Print and shaded views of the part. All mm, measured from the part's lowest x, y and z. A direction names the side the tool comes from. Round coordinates to 2 decimals unless told otherwise and drop trailing zeros. Loops run counter-clockwise (first coordinate to the right, second up) from the corner with the lowest first, then second, coordinate; pieces in that order, holes last. Notation, with made-up numbers: (-13, 64.25) -> (11, 64.25) arc R26 cw to (11, 86.25) -> close; hole circle Ø10 at (-20.75, 41). An arc over 180 degrees is marked (long way). Use a Markdown table: item, result.
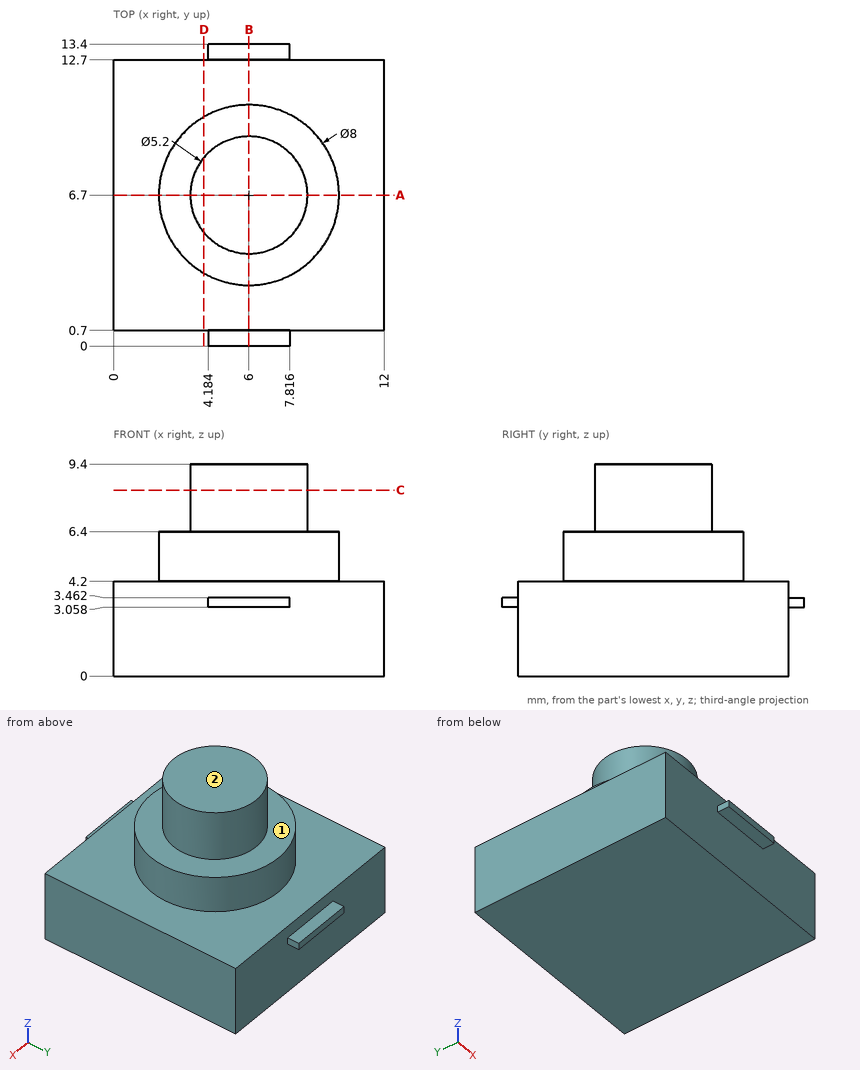
Q1. Band-saw the part on D-D, the plane x = 4. Give the cut face in (y, z).
Results list:
| item | result |
|---|---|
| outline | (0.7, 0) -> (12.7, 0) -> (12.7, 4.2) -> (10.16, 4.2) -> (10.16, 6.4) -> (8.36, 6.4) -> (8.36, 9.4) -> (5.04, 9.4) -> (5.04, 6.4) -> (3.24, 6.4) -> (3.24, 4.2) -> (0.7, 4.2) -> close |
Q2. Band-saw the part on A-A, the plane y = 6.7. Give the cut face in (x, z).
Results list:
| item | result |
|---|---|
| outline | (0, 0) -> (12, 0) -> (12, 4.2) -> (10, 4.2) -> (10, 6.4) -> (8.6, 6.4) -> (8.6, 9.4) -> (3.4, 9.4) -> (3.4, 6.4) -> (2, 6.4) -> (2, 4.2) -> (0, 4.2) -> close |
Q3. Band-saw the part on C-C, the plane z = 8.25. Give the cut face in (x, y), plus the area to 3 significant figures.
Results list:
| item | result |
|---|---|
| outline | circle Ø5.2 at (6, 6.7) |
| area | 21.2 mm² |
Q4. Tool access for the marked faces 1 and 2: list every direction of +Z, -Z, +X, -X, +Y, -Y with a clear straight run to the whole face (end or side of a thin tool).
Results list:
| item | result |
|---|---|
| face 1 | +Z |
| face 2 | +Z, +X, -X, +Y, -Y |
Q5. Flat gauge pins, fed straight in: pin 1 (1.3 mm diameter, centred on x = 4, z = 2, fed in from +Y); pin 2 (2 mm diameter, centred on x = 3, z = 1.5, fed in from -Y); pin 3 (0.6 mm diameter, centred on x = 6, y = 0, fed in from +Z). Where does each tip first touch, or does it go through?
Results list:
| item | result |
|---|---|
| pin 1 | stops at y = 12.7 |
| pin 2 | stops at y = 0.7 |
| pin 3 | stops at z = 3.46 |
Q6. Band-saw the part on B-B, the plane x = 6. Give the cut face in (y, z).
Results list:
| item | result |
|---|---|
| outline | (0, 3.06) -> (0.7, 3.06) -> (0.7, 0) -> (12.7, 0) -> (12.7, 3.06) -> (13.4, 3.06) -> (13.4, 3.46) -> (12.7, 3.46) -> (12.7, 4.2) -> (10.7, 4.2) -> (10.7, 6.4) -> (9.3, 6.4) -> (9.3, 9.4) -> (4.1, 9.4) -> (4.1, 6.4) -> (2.7, 6.4) -> (2.7, 4.2) -> (0.7, 4.2) -> (0.7, 3.46) -> (0, 3.46) -> close |
Q7. Drill centre lines: L1, parallel to Y at x = 7, z = 1.75; L2, parallel to Z at x = 8.75, y = 1.75; L3, parallel to Z at x = 8, y = 3.5. Where is each one in solid material? Low to high. Write a range as from..to.
Results list:
| item | result |
|---|---|
| L1 | y = 0.7..12.7 |
| L2 | z = 0..4.2 |
| L3 | z = 0..6.4 |
